Input: part model. Units: mm. Frame: model coordinates. A direction names the side the tool comes from. Coordinates: 2 decimals unless noted, no trailing zeros. Order: outer loops, then holes, each group sorted by start corner. A loop starts at its lowest first (then second) coordinate and runs counter-clockwise, first axis right, second up.
Autodesk Inventor part; units mm, degrees
ref_plane "YZ Plane" through (0, 0, 0) normal (1, 0, 0) x (0, 1, 0)
ref_plane "XZ Plane" through (0, 0, 0) normal (0, 1, 0) x (-1, 0, 0)
ref_plane "XY Plane" through (0, 0, 0) normal (0, 0, 1) x (1, 0, 0)
sketch "Sketch1" plane through (0, 0, 0) normal (0, 0, 1) x (1, 0, 0)
  line L0 (-0.7, 9.467) -> (-2.4, 9.467)
  line L1 (-2.4, 9.467) -> (-20.6434, -8.7764)
  line L2 (-20.6434, -8.7764) -> (-20.6434, -10.1764)
  line L3 (-20.6434, -10.1764) -> (-16.3229, -14.4968)
  line L4 (-16.3229, -14.4968) -> (-3.2414, -1.4153)
  line L5 (-22.6434, -8.2308) -> (-3.3393, 11.0732)
  line L6 (-22.6434, -8.2308) -> (-22.6434, -11.0308)
  line L7 (-27.2408, -15.6282) -> (-22.6434, -11.0308)
  line L8 (-30.0408, -15.6282) -> (-31.2428, -16.8303)
  line L9 (-31.2428, -16.8303) -> (-23.7475, -24.3256)
  line L10 (-16.6765, -17.2545) -> (-19.9434, -13.9876)
  line L11 (-19.9434, -13.9876) -> (-25.9538, -19.998)
  line L12 (-25.9538, -19.998) -> (-22.6869, -23.2649)
  line L13 (-23.7475, -24.3256) -> (-22.6869, -23.2649)
  line L14 (-16.6765, -17.2545) -> (-1.4029, -1.981)
  line L15 (-30.0408, -15.6282) -> (-27.2408, -15.6282)
  line L16 (3.3393, 11.0732) -> (-3.3393, 11.0732)
  line L17 (-0.7, 3.467) -> (-0.7, 9.467)
  line L18 (0, 12.3968) -> (0, -27.803) construction
  line L19 (0.7, 9.467) -> (2.4, 9.467)
  line L20 (2.4, 9.467) -> (20.6434, -8.7764)
  line L21 (20.6434, -8.7764) -> (20.6434, -10.1764)
  line L22 (20.6434, -10.1764) -> (16.3229, -14.4968)
  line L23 (16.3229, -14.4968) -> (3.2414, -1.4153)
  line L24 (22.6434, -8.2308) -> (3.3393, 11.0732)
  line L25 (22.6434, -8.2308) -> (22.6434, -11.0308)
  line L26 (27.2408, -15.6282) -> (22.6434, -11.0308)
  line L27 (30.0408, -15.6282) -> (31.2428, -16.8303)
  line L28 (31.2428, -16.8303) -> (23.7475, -24.3256)
  line L29 (16.6765, -17.2545) -> (19.9434, -13.9876)
  line L30 (19.9434, -13.9876) -> (25.9538, -19.998)
  line L31 (25.9538, -19.998) -> (22.6869, -23.2649)
  line L32 (23.7475, -24.3256) -> (22.6869, -23.2649)
  line L33 (16.6765, -17.2545) -> (1.4029, -1.981)
  line L34 (30.0408, -15.6282) -> (27.2408, -15.6282)
  line L35 (0.7, 3.467) -> (0.7, 9.467)
  arc A0 (1.4029, -1.981) -> (-1.4029, -1.981) centre (0, 0) ccw
  arc A1 (3.2414, -1.4153) -> (0.7, 3.467) centre (0, 0) ccw
  arc A2 (-0.7, 3.467) -> (-3.2414, -1.4153) centre (0, 0) ccw
  dimension "d77" = 1.8
  dimension "d83" = 27.3
  dimension "d84" = 135
  dimension "d87" = 2.8
  dimension "d88" = 135
  dimension "d89" = 2.8
  dimension "d90" = 1.7
  dimension "d93" = 4
  dimension "d94" = 1.5
  dimension "d96" = 8.5
  dimension "d100" = 1.4
  dimension "d101" = 2.2
  dimension "d102" = 2
  dimension "d103" = 1.7
  dimension "d104" = 10.6
  dimension "d106" = 135
  dimension "d107" = 25.8
  dimension "d108" = 18.5
  dimension "d109" = 21.6
  dimension "d110" = 6
  dimension "d111" = 0.7
  dimension "d112" = 1.7
extrude "Extrusion1" add sketch "Sketch1" against normal blind 26
properties part number "BRA-12 ESCUADRA UNIÓN 45 10 mm"
Item 1: Cut plane A-A on x = 8. Return loops of the section in (y, z).
Response values:
outline: (-8.58, -26) - (-6.17, -26) - (-6.17, 0) - (-8.58, 0) - close; (3.87, -26) - (6.41, -26) - (6.41, 0) - (3.87, 0) - close
Item 2: Ray query, probe 1 along X at (y, z) = (5, -15); probe 2 along X at (y, z) = (0, -17.5); probe 3 along X at (y, z) = (-3, -14.5). Return the intervals inside material, ascending.
Response values:
probe 1: x = -9.41 to -6.87, -0.7 to 0.7, 6.87 to 9.41
probe 2: x = -14.41 to -11.87, -3.54 to -2.43, 2.43 to 3.54, 11.87 to 14.41
probe 3: x = -17.41 to -14.87, -4.83 to -2.42, 2.42 to 4.83, 14.87 to 17.41
Item 3: Access query for faces 1 (the face through (29, -15.628, -13)), 2 (the face through (-22.643, -10, -13)), 3 (the face through (24.34, -21.61, -12.82)). Directions: +Z, -Z, +X, -X, +Y, -Y. A direction counts if a zero-diameter tool reaches every point of the face in a straight line with its end or side. Return the directions, or none.
Response values:
face 1: +Z, -Z, +X, +Y
face 2: +Z, -Z, -X, +Y
face 3: +Z, -Z
Item 4: Draft query along X for faces 4 (the face through (13.126, 1.286, -12.818)), 5 (the face through (-2.5, -2.6, -26)), 6 (the face through (-30.63, -16.22, -12.82)), 7 (the face through (9.147, -9.725, -12.818)). Return one class per face: pulls with the +X half, pulls with the -X half, needs draft (parallel to the pull), parting line crosses it, or undercut.
Response values:
face 4: pulls with the +X half
face 5: needs draft
face 6: pulls with the -X half
face 7: undercut
Item 5: Cut plane C-C on z = -14.25. Count the separate pieces of the cut face and the enclosed holes in it, then the cut area to 3 significant figures.
Response values:
separate pieces: 1
enclosed holes: 2
area: 341 mm2
Item 6: Cut plane B-B on y = 0. Return loops of the section in (x, z).
Response values:
outline: (-14.41, -26) - (-11.87, -26) - (-11.87, 0) - (-14.41, 0) - close; (-3.54, -26) - (-2.43, -26) - (-2.43, 0) - (-3.54, 0) - close; (2.43, -26) - (3.54, -26) - (3.54, 0) - (2.43, 0) - close; (11.87, -26) - (14.41, -26) - (14.41, 0) - (11.87, 0) - close
Item 7: Cut plane D-D on y = -19. Return loops of the section in (x, z), then the cut area to 3 significant figures.
Response values:
outline: (-29.07, -26) - (-24.96, -26) - (-24.96, 0) - (-29.07, 0) - close; (24.96, -26) - (29.07, -26) - (29.07, 0) - (24.96, 0) - close
area: 214 mm2
Item 8: Pin query (flat end, axial travel): pin 1 Ø1 at (y, z) = (0.5, -13) entering from +X; pin 2 Ø10 at (x, y) = (20.5, -9) entering from -Z; pin 3 Ø0.8 at (y, z) = (-9.5, -14.5) entering from -X; pin 4 Ø1.4 at (y, z) = (-10, -18.5) entering from +X. Return the tip coordinate at first contact, or that it passes through.
Response values:
pin 1: stops at x = 14.41
pin 2: stops at z = -26
pin 3: stops at x = -22.64
pin 4: stops at x = 22.64
